Check sheet for the modelled part. Datum: model origin and axes. Units: mm. Face numbers are marked on the shaded views. A direction names the side the tool comes from. Coordinates: 2 decimals unless noted, no trailing zeros. Loops run counter-clockwise (first coordinate to the right, second up) from the corner with the lowest first, then second, coordinate; pieces in that order, holes last. Notation, with made-up numbers: M 42.5,58.25 L 92.5,58.25 A15 ccw 92.5,64.25 Z; hole C 18,-21.75 d1. An arc over 180 degrees is marked long. Write each question's results on one line, items separated by ' | '. Start each with the question number.
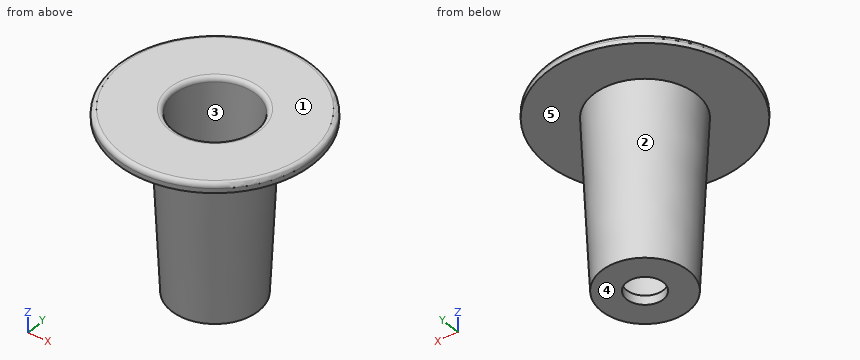
from build123d import *

# Parameters (mm, degrees)
FILLET_R = 1


with BuildPart() as part:
    # Sketch → Revolution (revolve)
    with BuildSketch(Plane.XZ):
        Polygon((9, 39.5), (21.5, 39.5), (21.5, 37.5), (11.25, 37.5), (9.5, 0), (4, 0), (4, 2), (7.25, 2), align=None)
    revolve(axis=Axis((0, 0, 0), (0, 0, 1)))

    # Fillet
    fillet_edges = [part.edges().sort_by_distance(p)[0] for p in [
        (-21.5, 0, 39.5),
        (-9, 0, 39.5),
    ]]
    fillet(fillet_edges, radius=FILLET_R)


solid = part.part
1) Section check C-C (z = 9). Enter the section's corners in (x, y).
2) Section check A-A (y = 0). Enter the section's corners in (x, z).
3) Gauge pin test, flat ends, axial feed: P1, Ø3, axis at x = -6.5, z = 7, coming from the +Y side; P2, Ø3, axis at x = -9, z = 26, coming from the +Y side; P3, Ø6, axis at x = 7, z = 11, coming from the -Y side. Record the tip position at first contact, or that the pin passes through.
4) Section check D-D (z = 23). Enter the section's corners in (x, y), then the cut area to 3 significant figures.
5) Set-up check for the marked faces 4 and 5: record each of +Z, -Z, +X, -X, +Y, -Y from which the full face is reachable in a straight line by a thin tool's end or side.
6) Thickness scan on probe 1 along Z at (x, y) = (-6, 14); probe 2 along Y at (x, z) = (0, 1.5); probe 3 along X at (y, z) = (-1, 29). Record the ranges inside material, lowest first.
7) Release check for a two-part mould opening along X. For the marked faces 1, 2 and 3 record: +X half, -X half, draft (parallel to the pull), parting line (faces both ways), or undercut.
Return value:
1) outline: C 0,0 d19.84; hole C 0,0 d15.15
2) outline: M -21.5,37.5 L -11.25,37.5 L -9.5,0 L -4,0 L -4,2 L -7.25,2 L -8.96,38.55 A1 ccw -9.95,39.5 L -20.5,39.5 A1 ccw -21.5,38.5 Z; M 4,0 L 9.5,0 L 11.25,37.5 L 21.5,37.5 L 21.5,38.5 A1 ccw 20.5,39.5 L 9.95,39.5 A1 ccw 8.96,38.55 L 7.25,2 L 4,2 Z
3) P1: stops at y = 8.46 | P2: stops at y = 7.65 | P3: stops at y = -9.19
4) outline: C 0,0 d21.15; hole C 0,0 d16.46 | area: 138 mm2
5) face 4: -Z, +X, -X, +Y, -Y | face 5: -Z
6) probe 1: z = 37.5 to 39.5 | probe 2: y = -9.57 to -4, 4 to 9.57 | probe 3: x = -10.81 to -8.45, 8.45 to 10.81
7) face 1: draft | face 2: parting line | face 3: undercut
